The listing builds one solid part. Answer for the finished solid, in the listing's coordinates (mm). Round coordinates to 2 decimals unless told otherwise and drop trailing zeros. Loops run counter-clockwise (first coordinate to the right, second up) from the corner with the lowest first, then second, coordinate; pieces in that order, holes last. Notation, with made-up numbers: (89.5, -31) -> (140.5, -31) arc R20 cw to (140.5, -4) -> close; hole circle Ø3 at (85, 67.5). An arc over 180 degrees is marked (long way). One line per question, with ' | ' between items.
from build123d import *

# Parameters (mm, degrees)
SKETCH_W     = 57.26
SKETCH_H     = 40.62
PAD_DEPTH    = 2.2
SKETCH001_W  = 60.26
SKETCH001_H  = 42.72
PAD001_DEPTH = 2.2
SKETCH002_W  = 0.1
SKETCH002_H  = 10.6
PAD002_DEPTH = 1.7
SKETCH003_W  = 10.6
SKETCH003_H  = 0.1
PAD003_DEPTH = 17.4
SKETCH004_W  = 49.66
SKETCH004_H  = 37.42
PAD004_DEPTH = 1
FILLET_R     = 0.5
SKETCH005_W  = 10
SKETCH005_H  = 0.1
PAD005_DEPTH = 13.8
FILLET001_R  = 0.5
SKETCH006_W  = 10
SKETCH006_H  = 0.1
PAD006_DEPTH = 3
POCKET_DEPTH = 0.1
FILLET002_R  = 0.5
FILLET003_R  = 0.5


with BuildPart() as part:
    # Sketch → Pad (new body)
    with BuildSketch(Plane.XY):
        Rectangle(SKETCH_W, SKETCH_H)
    extrude(amount=PAD_DEPTH)

    # Sketch001 (on Face6 of Pad) → Pad001 (join)
    with BuildSketch(Plane.XY.offset(2.2)):
        Rectangle(SKETCH001_W, SKETCH001_H)
    extrude(amount=-PAD001_DEPTH)

    # Sketch002 (on Face5 of Pad001) → Pad002 (join)
    with BuildSketch(Plane(origin=(0, 0, 0), x_dir=(1, 0, 0), z_dir=(0, 0, -1))):
        with Locations((30.08, 0)):
            Rectangle(SKETCH002_W, SKETCH002_H)
    extrude(amount=PAD002_DEPTH)

    # Sketch003 (on Face10 of Pad002) → Pad003 (join)
    with BuildSketch(Plane(origin=(30.03, 0, 0), x_dir=(0, -1, 0), z_dir=(-1, 0, 0))):
        with Locations((0, -1.65)):
            Rectangle(SKETCH003_W, SKETCH003_H)
    extrude(amount=PAD003_DEPTH)

    # Sketch004 (on Face8 of Pad003) → Pad004 (join)
    with BuildSketch(Plane.XY.offset(2.2)):
        with Locations((-2.2, 0)):
            Rectangle(SKETCH004_W, SKETCH004_H)
    extrude(amount=-PAD004_DEPTH)

    # Fillet
    fillet_edges = [part.edges().sort_by_distance(p)[0] for p in [
        (12.63, -5.3, -1.65),
        (12.63, 5.3, -1.65),
    ]]
    fillet(fillet_edges, radius=FILLET_R)

    # Sketch005 (on Face1 of Fillet) → Pad005 (join)
    with BuildSketch(Plane(origin=(0, 5.3, 0), x_dir=(-1, 0, 0), z_dir=(0, 1, 0))):
        with Locations((-24.13, -1.65)):
            Rectangle(SKETCH005_W, SKETCH005_H)
    extrude(amount=PAD005_DEPTH)

    # Fillet001
    fillet001_edges = [part.edges().sort_by_distance(p)[0] for p in [
        (19.13, 19.1, -1.65),
        (29.13, 19.1, -1.65),
    ]]
    fillet(fillet001_edges, radius=FILLET001_R)

    # Sketch006 (on Face16 of Fillet001) → Pad006 (join)
    with BuildSketch(Plane.XZ.offset(5.3)):
        with Locations((25.13, -1.65)):
            Rectangle(SKETCH006_W, SKETCH006_H)
    extrude(amount=PAD006_DEPTH)

    # Sketch007 (on Face33 of Pad006) → Pocket (cut)
    with BuildSketch(Plane.XY.offset(2.2)):
        with BuildLine():
            ThreePointArc((26.23, 10), (25.73, 10.5), (25.23, 10))
            Line((25.23, 10), (25.23, -10))
            ThreePointArc((25.23, -10), (25.73, -10.5), (26.23, -10))
            Line((26.23, -10), (26.23, 10))
        make_face()
    extrude(amount=-POCKET_DEPTH, mode=Mode.SUBTRACT)

    # Fillet002
    fillet002_edges = [part.edges().sort_by_distance(p)[0] for p in [
        (20.13, -8.3, -1.65),
    ]]
    fillet(fillet002_edges, radius=FILLET002_R)

    # Fillet003
    fillet003_edges = [part.edges().sort_by_distance(p)[0] for p in [
        (30.13, -8.3, -1.65),
    ]]
    fillet(fillet003_edges, radius=FILLET003_R)


solid = part.part
Q1. Given pin 1 Ø8 at (x, y) = (-14, 3.5) entering from -Z; pin 2 Ø1.8 at (y, z) = (-0.5, -1) entering from -X; pin 3 Ø0.5 at (x, z) = (29.5, -1) entering from +Y, each flat-ended and moving along its own axis, determine where each tip first touches the part or whether it passes through.
Numbers:
pin 1: z = 0 | pin 2: x = 12.63 | pin 3: through
Q2. A cutting plane is placed at C-C on x = -5.5. Give the vertices of the cut face in (y, z), plus the area to 3 significant figures.
Numbers:
outline: (-21.36, 0) -> (21.36, 0) -> (21.36, 2.2) -> (-21.36, 2.2) -> close | area: 94.0 mm^2
Q3. A cutting plane is placed at A-A on y = 18. Give the vertices of the cut face in (x, z), plus the area to 3 significant figures.
Numbers:
outline: (-30.13, 0) -> (30.13, 0) -> (30.13, 2.2) -> (-30.13, 2.2) -> close; (19.13, -1.7) -> (29.13, -1.7) -> (29.13, -1.6) -> (19.13, -1.6) -> close | area: 134 mm^2
Q4. Find the intervals of material crossed by line 1 (Z direction, x = 3, y = 12), in increasing order. Write a range as from..to.
Numbers:
line 1: 0..2.2
Q5. A cutting plane is placed at B-B on z = -0.7. Give the vertices of the cut face in (x, y), plus the area to 3 significant figures.
Numbers:
outline: (30.03, -5.3) -> (30.13, -5.3) -> (30.13, 5.3) -> (30.03, 5.3) -> close | area: 1.06 mm^2
